Could you check a few things on this model? Use its own coordinates, in mm. Face numbers are marked on the shaded views. A direction names the side the tool comes from. Give positions to 0.01 mm unless a question says otherwise; leave off trailing zeros. Loops run counter-clockwise (first coordinate to the right, second up) from the corner with the lowest first, then second, coordinate; pieces in that order, holes last. Notation, with made-up numbers: (42, 55) -> (77, 55) arc R16 cw to (77, 67) -> close; hole circle Ø4 at (12, -24.75). An arc over 180 degrees is marked (long way). Put each result on its own line as item: value.
```python
from build123d import *

# Parameters (mm, degrees)
SKETCH2_R           = 2.5
BOSS_EXTRUDE1_DEPTH = 7
SKETCH3_W           = 6
SKETCH3_H           = 1.8
CUT_EXTRUDE1_DEPTH  = 7
SKETCH4_R           = 2
CUT_EXTRUDE2_DEPTH  = 2


with BuildPart() as part:
    # Sketch2 → Boss-Extrude1 (new body)
    with BuildSketch(Plane.XY):
        with BuildLine():
            Line((-4, 0), (-4, 10))
            Line((-4, 10), (4, 10))
            Line((4, 10), (4, 0))
            ThreePointArc((4, 0), (0, -4), (-4, 0))
        make_face()
        Circle(SKETCH2_R, mode=Mode.SUBTRACT)
    extrude(amount=BOSS_EXTRUDE1_DEPTH)

    # Sketch3 → Cut-Extrude1 (cut)
    with BuildSketch(Plane.XY.offset(7)):
        with Locations((0, 8)):
            Rectangle(SKETCH3_W, SKETCH3_H)
    extrude(amount=-CUT_EXTRUDE1_DEPTH, mode=Mode.SUBTRACT)

    # Sketch4 → Cut-Extrude2 (cut)
    with BuildSketch(Plane(origin=(0, 10, 0), x_dir=(1, 0, 0), z_dir=(0, 1, 0))):
        with Locations((0, -3.5)):
            Circle(SKETCH4_R)
    extrude(amount=-CUT_EXTRUDE2_DEPTH, mode=Mode.SUBTRACT)


solid = part.part
```
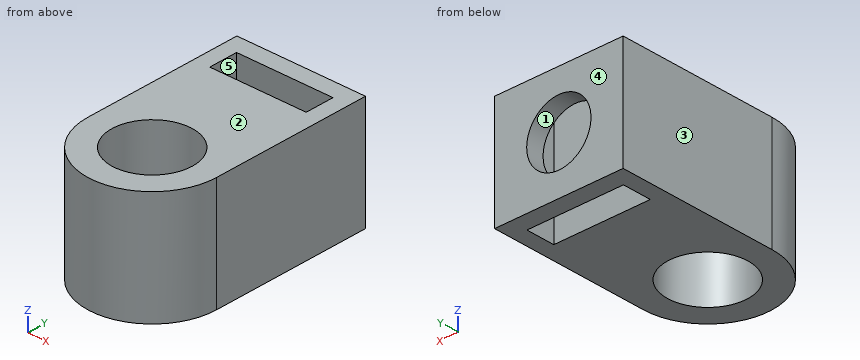
1. If we section it at B-B (y = 2): List the corners of the cut face in (x, z) for me, then the cut area to 3 significant figures.
Recorded:
outline: (-4, 0) -> (-1.5, 0) -> (-1.5, 7) -> (-4, 7) -> close; (1.5, 0) -> (4, 0) -> (4, 7) -> (1.5, 7) -> close
area: 35.0 mm^2
2. If we section it at D-D (z = 3.5): List the corners of the cut face in (x, y) for me, then the cut area to 3 significant figures.
Recorded:
outline: (-4, 0) arc R4 ccw to (4, 0) -> (4, 10) -> (2, 10) -> (2, 8.9) -> (3, 8.9) -> (3, 7.1) -> (-3, 7.1) -> (-3, 8.9) -> (-2, 8.9) -> (-2, 10) -> (-4, 10) -> close; hole circle Ø5 at (0, 0)
area: 70.3 mm^2
3. If we section it at A-A (x = 0): List the corners of the cut face in (y, z) for me, then the cut area to 3 significant figures.
Recorded:
outline: (-4, 0) -> (-2.5, 0) -> (-2.5, 7) -> (-4, 7) -> close; (2.5, 0) -> (7.1, 0) -> (7.1, 7) -> (2.5, 7) -> close; (8.9, 0) -> (10, 0) -> (10, 1.5) -> (8.9, 1.5) -> close; (8.9, 5.5) -> (10, 5.5) -> (10, 7) -> (8.9, 7) -> close
area: 46.0 mm^2
4. If we section it at C-C (z = 6.25): List the corners of the cut face in (x, y) for me, then the cut area to 3 significant figures.
Recorded:
outline: (-4, 0) arc R4 ccw to (4, 0) -> (4, 10) -> (-4, 10) -> close; hole (-3, 7.1) -> (3, 7.1) -> (3, 8.9) -> (-3, 8.9) -> close; hole circle Ø5 at (0, 0)
area: 74.7 mm^2
5. I need wall thicknesses on line 1 (Y direction, x = 0, z = 6); line 2 (X direction, y = 9.7, z = 3.5); line 3 (Z direction, x = 0, y = 9.6). Which ranges of each line are inside material? Lowest first, please.
Recorded:
line 1: y = -4 to -2.5, 2.5 to 7.1, 8.9 to 10
line 2: x = -4 to -2, 2 to 4
line 3: z = 0 to 1.5, 5.5 to 7
6. Thinking about a two-plate mould opening in Z: for the marked faces 1, 2 and 3, which applies, pulls with the +Z half, pulls with the -Z half, needs draft (parallel to the pull), parting line crosses it, or undercut?
Recorded:
face 1: undercut
face 2: pulls with the +Z half
face 3: needs draft
7. For the marked faces 4 and 5, which set-ups out of +Z, -Z, +X, -X, +Y, -Y let a thin tool reach every point of the face, with its end or its side?
Recorded:
face 4: +Z, -Z, +X, -X, +Y
face 5: +Z, -Z
